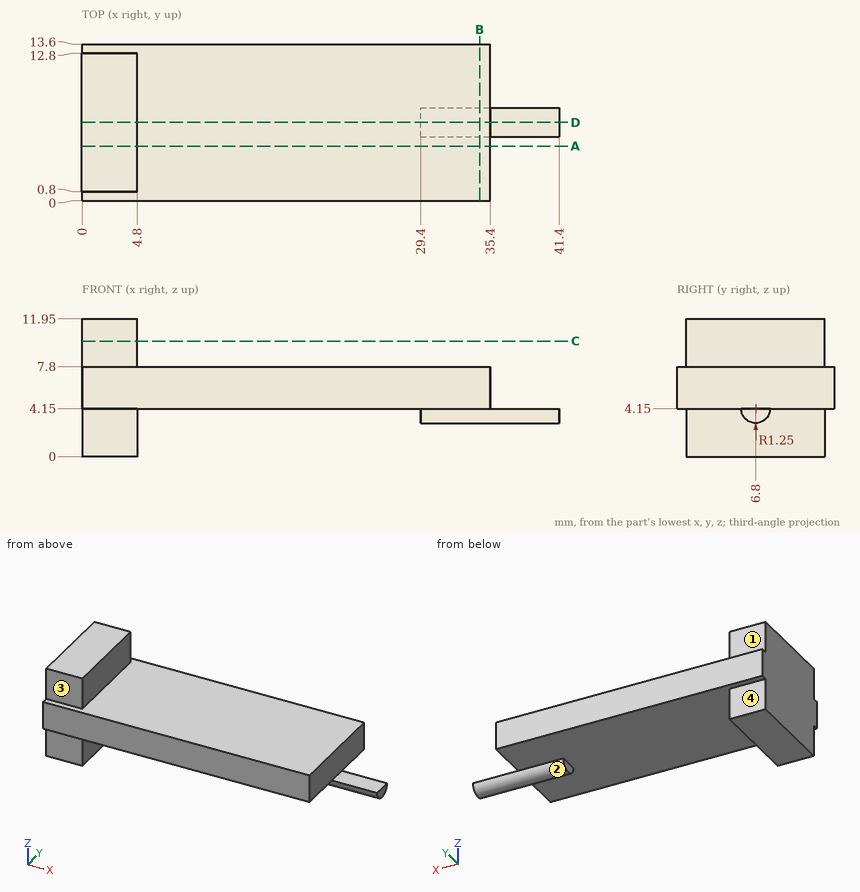
For this review, use the dimensioned drawing (mm, ordinates from the lowest corner) and the shaded views. A direction names the side the tool comes from. Coordinates: 2 decimals unless noted, no trailing zeros. Loops run counter-clockwise (first coordinate to the right, second up) from the corner with the lowest first, then second, coordinate; pieces in that order, holes last. Notation, with made-up numbers: (-0.5, -12.5) -> (19.5, -12.5) arc R26 ccw to (19.5, 13.5) -> close; hole circle Ø9 at (11, 25.5). An arc over 180 degrees is marked (long way). Return JSON: item names as keys, results as strings. Group by question number.
(1) Consider section B-B, the plane x = 34.5. Give the boundary of the cut face in (y, z).
(2) To check wall thickness, follow L1, parallel to Z at x = 6, y = 5.25; L2, parallel to X at y = 11.25, z = 5; L3, parallel to X at y = 4, z = 11. State the ranges of each line that lie inside material, in increasing order.
(3) Tool access review of the marked faces 1, 2, 3 and 4: name each direction out of +Z, -Z, +X, -X, +Y, -Y from which nothing blocks a thin tool from reaching the whole face with its end or side.
(4) Consider section C-C, the plane z = 10. Give the boundary of the cut face in (x, y).
(5) Consider section D-D, the plane y = 6.8. Give the boundary of the cut face in (x, z), plus the area to 3 significant figures.
(6) For pin 1 Ø1.5 at (x, y) = (30, 2) entering from -Z; pin 2 Ø8 at (x, y) = (31.5, 9) entering from +Z; pin 3 Ø1.8 at (y, z) = (7.5, 5.5) entering from +X, all flat-tipped, find the tip position at first contact; note any pin that passes through.
(7) Consider section A-A, the plane y = 4.75. Give the boundary of the cut face in (x, z).
Results below:
{
 "1": {"outline": "(0, 4.15) -> (5.55, 4.15) arc R1.25 ccw to (8.05, 4.15) -> (13.6, 4.15) -> (13.6, 7.8) -> (0, 7.8) -> close"},
 "2": {"L1": "z = 4.15 to 7.8", "L2": "x = 0 to 35.4", "L3": "x = 0 to 4.8"},
 "3": {"face 1": "+Z, +X, -X, +Y", "face 2": "-Z, +X", "face 3": "+Z, +X, -X, -Y", "face 4": "-Z, +X, -X, +Y"},
 "4": {"outline": "(0, 0.8) -> (4.8, 0.8) -> (4.8, 12.8) -> (0, 12.8) -> close"},
 "5": {"outline": "(0, 0) -> (4.8, 0) -> (4.8, 4.15) -> (29.4, 4.15) -> (29.4, 2.9) -> (41.4, 2.9) -> (41.4, 4.15) -> (35.4, 4.15) -> (35.4, 7.8) -> (4.8, 7.8) -> (4.8, 11.95) -> (0, 11.95) -> close", "area": "184 mm2"},
 "6": {"pin 1": "stops at z = 4.15", "pin 2": "stops at z = 7.8", "pin 3": "stops at x = 35.4"},
 "7": {"outline": "(0, 0) -> (4.8, 0) -> (4.8, 4.15) -> (35.4, 4.15) -> (35.4, 7.8) -> (4.8, 7.8) -> (4.8, 11.95) -> (0, 11.95) -> close"}
}
